Design review of the part built by this model. Coordinates are the model's own, in mm. A direction names the side the tool comes from. Coordinates: 2 decimals unless noted, no trailing zeros. Loops run counter-clockwise (first coordinate to the right, second up) from the corner with the lowest first, then second, coordinate; pieces in that order, holes last.
from build123d import *

# Parameters (mm, degrees)
SKETCH1_W            = 165
SKETCH1_H            = 90
BOSS_EXTRUDE1_DEPTH  = 3
SKETCH2_W            = 5
SKETCH2_H            = 38
BOSS_EXTRUDE3_DEPTH  = 38
FILLET1_R            = 5
SKETCH3_R            = 2.5
BOSS_EXTRUDE4_DEPTH  = 5
SKETCH4_W            = 3
SKETCH4_H            = 20
BOSS_EXTRUDE5_DEPTH  = 23
SKETCH5_W            = 76
SKETCH5_H            = 20
BOSS_EXTRUDE6_DEPTH  = 3
FILLET3_R            = 3
FILLET4_R            = 3
SKETCH8_W            = 10
SKETCH8_H            = 22
CUT_EXTRUDE1_DEPTH   = 10
FILLET10_R           = 5
SKETCH9_W            = 10
SKETCH9_H            = 22
CUT_EXTRUDE2_DEPTH   = 10
FILLET11_R           = 5
SKETCH10_W           = 165
SKETCH10_H           = 6
BOSS_EXTRUDE9_DEPTH  = 3
FILLET13_R           = 4
SKETCH11_R           = 2.5
BOSS_EXTRUDE10_DEPTH = 5
FILLET14_R           = 2


with BuildPart() as part:
    # Sketch1 → Boss-Extrude1 (new body)
    with BuildSketch(Plane(origin=(0, 0, 0), x_dir=(1, 0, 0), z_dir=(0, 1, 0))):
        with Locations((82.5, 45)):
            Rectangle(SKETCH1_W, SKETCH1_H)
    extrude(amount=BOSS_EXTRUDE1_DEPTH)

    # Sketch2 → Boss-Extrude3 (add)
    with BuildSketch(Plane(origin=(0, 3, 0), x_dir=(1, 0, 0), z_dir=(0, 1, 0))):
        with Locations((15, 45)):
            Rectangle(SKETCH2_W, SKETCH2_H)
        with Locations((150, 45)):
            Rectangle(SKETCH2_W, SKETCH2_H)
    extrude(amount=BOSS_EXTRUDE3_DEPTH)

    # Fillet1
    fillet1_edges = [part.edges().sort_by_distance(p)[0] for p in [
        (12.5, 3, -45),
        (15, 3, -26),
        (17.5, 3, -45),
        (15, 3, -64),
        (150, 3, -64),
        (147.5, 3, -45),
        (150, 3, -26),
        (152.5, 3, -45),
    ]]
    fillet(fillet1_edges, radius=FILLET1_R)

    # Sketch3 → Boss-Extrude4 (add)
    with BuildSketch(Plane(origin=(0, 41, 0), x_dir=(1, 0, 0), z_dir=(0, 1, 0))):
        with Locations(Location((15, 57, 0), (0, 0, 180))):
            Circle(SKETCH3_R)
        with Locations(Location((15, 33, 0), (0, 0, 180))):
            Circle(SKETCH3_R)
        with Locations(Location((150, 57, 0), (0, 0, 180))):
            Circle(SKETCH3_R)
        with Locations(Location((150, 33, 0), (0, 0, 180))):
            Circle(SKETCH3_R)
    extrude(amount=BOSS_EXTRUDE4_DEPTH)

    # Sketch4 → Boss-Extrude5 (add)
    with BuildSketch(Plane(origin=(0, 3, 0), x_dir=(1, 0, 0), z_dir=(0, 1, 0))):
        with Locations((119, 45)):
            Rectangle(SKETCH4_W, SKETCH4_H)
        with Locations((46, 45)):
            Rectangle(SKETCH4_W, SKETCH4_H)
    extrude(amount=BOSS_EXTRUDE5_DEPTH)

    # Sketch5 → Boss-Extrude6 (add)
    with BuildSketch(Plane(origin=(0, 26, 0), x_dir=(1, 0, 0), z_dir=(0, 1, 0))):
        with Locations((82.5, 45)):
            Rectangle(SKETCH5_W, SKETCH5_H)
    extrude(amount=BOSS_EXTRUDE6_DEPTH)

    # Fillet3
    fillet3_edges = [part.edges().sort_by_distance(p)[0] for p in [
        (47.5, 3, -45),
        (47.5, 26, -45),
        (117.5, 3, -45),
        (117.5, 26, -45),
    ]]
    fillet(fillet3_edges, radius=FILLET3_R)

    # Fillet4
    fillet4_edges = [part.edges().sort_by_distance(p)[0] for p in [
        (120.5, 29, -45),
        (44.5, 29, -45),
    ]]
    fillet(fillet4_edges, radius=FILLET4_R)

    # Sketch8 → Cut-Extrude1 (cut)
    with BuildSketch(Plane.ZY.offset(-12.5)):
        with Locations((-45, 24.5)):
            Rectangle(SKETCH8_W, SKETCH8_H)
    extrude(amount=-CUT_EXTRUDE1_DEPTH, mode=Mode.SUBTRACT)

    # Fillet10
    fillet10_edges = [part.edges().sort_by_distance(p)[0] for p in [
        (15, 13.5, -50),
        (15, 35.5, -50),
        (15, 13.5, -40),
        (15, 35.5, -40),
    ]]
    fillet(fillet10_edges, radius=FILLET10_R - 0.0001)  # a hair under: the kernel refuses the full size

    # Sketch9 → Cut-Extrude2 (cut)
    with BuildSketch(Plane(origin=(152.5, 0, 0), x_dir=(0, 0, -1), z_dir=(1, 0, 0))):
        with Locations((45, 24.5)):
            Rectangle(SKETCH9_W, SKETCH9_H)
    extrude(amount=-CUT_EXTRUDE2_DEPTH, mode=Mode.SUBTRACT)

    # Fillet11
    fillet11_edges = [part.edges().sort_by_distance(p)[0] for p in [
        (150, 35.5, -40),
        (150, 13.5, -40),
        (150, 13.5, -50),
        (150, 35.5, -50),
    ]]
    fillet(fillet11_edges, radius=FILLET11_R - 0.0001)  # a hair under: the kernel refuses the full size

    # Sketch10 → Boss-Extrude9 (add)
    with BuildSketch(Plane.XZ):
        with Locations((82.5, -93)):
            Rectangle(SKETCH10_W, SKETCH10_H)
        with Locations((82.5, 3)):
            Rectangle(SKETCH10_W, SKETCH10_H)
    extrude(amount=-BOSS_EXTRUDE9_DEPTH)

    # Fillet13
    fillet13_edges = [part.edges().sort_by_distance(p)[0] for p in [
        (44.5, 3, -45),
        (120.5, 3, -45),
    ]]
    fillet(fillet13_edges, radius=FILLET13_R)

    # Sketch11 → Boss-Extrude10 (add)
    with BuildSketch(Plane(origin=(0, 41, 0), x_dir=(1, 0, 0), z_dir=(0, 1, 0))):
        with Locations(Location((150, 45, 0), (0, 0, 180))):
            Circle(SKETCH11_R)
        with Locations(Location((15, 45, 0), (0, 0, 180))):
            Circle(SKETCH11_R)
    extrude(amount=BOSS_EXTRUDE10_DEPTH)

    # Fillet14
    fillet14_edges = [part.edges().sort_by_distance(p)[0] for p in [
        (165, 3, -45),
        (82.5, 3, -96),
        (82.5, 3, 6),
        (0, 3, -45),
    ]]
    fillet(fillet14_edges, radius=FILLET14_R)


solid = part.part
Q1. For line 1 (X direction, y = 13, z = -61.5); line 2 (Y direction, x = 90.5, z = -53); line 3 (Y direction, x = 38, z = -65), list the stretches that pass through material, from the lowest coordinate up.
Q2. Machinability: for faces 4 (the flat face through (15, 24, -64)), 5 (the flat face through (15, 24, -26)), 6 (the flat face through (117.5, 14, -45)), which of the approach directions +Z, -Z, +X, -X, +Y, -Y give a long, thin tool a straight path to every point of the face, cutting with its end or side? Answer none if there is none.
Q3. The part is to be moulded in two halves that separate along X. For faces 1 (the cylindrical face through (15.04, 34.07, -48.5)), 2 (the cylindrical face through (15.54, 43.46, -47.44)), 3 (the flat face through (152.5, 24, -53)), say which applies: pulls with the +X half, pulls with the -X half, needs draft (parallel to the pull), parting line crosses it, or undercut.
Q4. Take a section at D-D, the plane z = -12.5. Write out the cut boundary in (x, y).
Q5. Take a section at A-A, the plane x = 70. Write out the cut boundary in (y, z), then the cut area to 3 significant figures.
Q6. Clearance check with flat-ended pins moving along their axes: pin 1 Ø3 at (x, y) = (145.5, 38.5) entering from -Z; pin 2 Ø12 at (y, z) = (13, -39) entering from +X; pin 3 Ø18.5 at (y, z) = (14, -42.5) entering from +X; pin 4 Ø21 at (y, z) = (15, -43.5) entering from -X. State where each tip first meets the part, or that it passes through.
Entries:
1. line 1: x = 12.5 to 17.5, 147.5 to 152.5
1. line 2: y = 0 to 3, 26 to 29
1. line 3: y = 0 to 3
2. face 4: -Z, +X, -X, +Y
2. face 5: +Z, +X, -X, +Y
2. face 6: +Z, -Z
3. face 1: needs draft
3. face 2: undercut
3. face 3: pulls with the +X half
4. outline: (0, 0) - (165, 0) - (165, 1) arc R2 ccw to (163, 3) - (2, 3) arc R2 ccw to (0, 1) - close
5. outline: (0, -96) - (1, -96) arc R2 ccw to (3, -94) - (3, 4) arc R2 ccw to (1, 6) - (0, 6) - close; (26, -55) - (29, -55) - (29, -35) - (26, -35) - close
5. area: 364 mm2
6. pin 1: passes through
6. pin 2: stops at x = 152.6
6. pin 3: stops at x = 153.7
6. pin 4: stops at x = 11.07
